Input: part model. Units: mm. Frame: model coordinates. Face numbers are marked on the shaded views. A direction names the side the tool comes from. Give positions to 0.01 mm unless a question says otherwise; leave off trailing zeros. Order: outer loops, then holes, each group sorted by start corner. A loop starts at its lowest first (then second) coordinate and runs counter-clockwise, first axis right, second up. Notation, with made-up numbers: (56.5, 64.5) - (69.5, 64.5) arc R11 ccw to (69.5, 76.5) - close; hole circle Ø2 at (-37, -38.75). An arc over 180 degrees is marked (long way). Use a Markdown table: item, result.
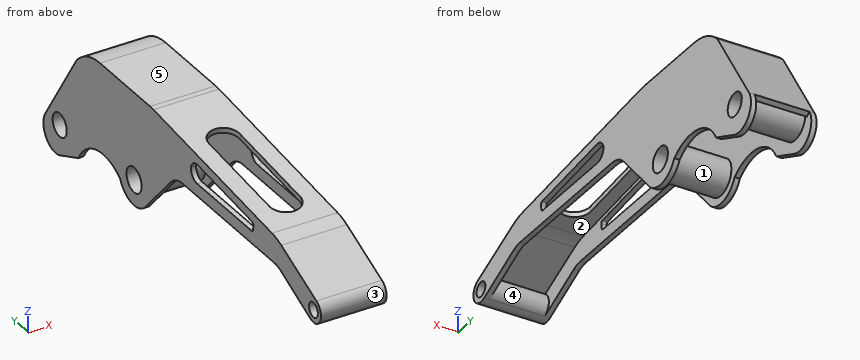
from build123d import *

# Parameters (mm, degrees)
F0_R        = 5.6533409101
F0_R_2      = 6.0582147302
F0_R_3      = 3.5468264326
F1_DEPTH    = 31.75
F2_T        = 2.54
F2_T3_DEPTH = 36.83
F4_DEPTH    = 25.4
F6_DEPTH    = 31.751
F7_T1_DEPTH = 2.54
F7_T3_DEPTH = 2.54
F8_R        = 1.27


# Not quite as in the source:
# - a fillet or chamfer that OpenCascade refuses, or shapes differently, is made with other operations: its cross-section is extruded or revolved along the edge and cut away or added
# - a shell that OpenCascade refuses in one call is made with other operations: the cavity is built on its own and cut out


with BuildPart() as f1:
    # F0 (on Right) → F1 (new body)
    with BuildSketch(Plane.YZ):
        with BuildLine():
            Line((-118.2969192854, 30.0553025028), (-146.4621126652, 17.7829619497))
            ThreePointArc((-146.4621126652, 17.7829619497), (-149.6721200055, 9.657338463), (-141.4359788777, 6.7425685756))
            Line((-141.4359788777, 6.7425685756), (-117.9046317908, 17.455203049))
            ThreePointArc((-117.9046317908, 17.455203049), (-115.3347971308, 18.3079832041), (-112.6425907814, 18.5966164392))
            Line((-112.6425907814, 18.5966164392), (-39.032237408, 18.5966164392))
            ThreePointArc((-39.032237408, 18.5966164392), (-33.875711062, 17.5026595222), (-29.6075339545, 14.4092520366))
            Line((-29.6075339545, 14.4092520366), (-10.1635284412, -7.1180392256))
            ThreePointArc((-10.1635284412, -7.1180392256), (1.0358015594, -12.3649063046), (11.2061193672, -5.3279153072))
            ThreePointArc((11.2061193672, -5.3279153072), (29.7519512617, -1.1293262164), (44.7507215315, -12.8174792531))
            Line((44.7507215315, -12.8174792531), (59.2673632914, -19.1176440206))
            ThreePointArc((59.2673632914, -19.1176440206), (70.5449926496, -16.490786447), (71.3009120761, -4.9359653548))
            Line((71.3009120761, -4.9359653548), (46.0699528524, 34.1704526075))
            ThreePointArc((46.0699528524, 34.1704526075), (37.5779975797, 40.2467968073), (27.3589767296, 42.3931602559))
            Line((27.3589767296, 42.3931602559), (-12.8688071267, 42.3931602559))
            ThreePointArc((-12.8688071267, 42.3931602559), (-14.2256285087, 42.3568949126), (-15.5785754345, 42.2482024399))
            Line((-15.5785754345, 42.2482024399), (-110.8605493232, 32.0248153133))
            ThreePointArc((-110.8605493232, 32.0248153133), (-114.6537287056, 31.3232183323), (-118.2969192854, 30.0553025028))
        make_face()
        with Locations((59.7972124815, -4.6163224615)):
            Circle(F0_R, mode=Mode.SUBTRACT)
        Circle(F0_R_2, mode=Mode.SUBTRACT)
        with Locations((-144.1483274102, 12.1720423922)):
            Circle(F0_R_3, mode=Mode.SUBTRACT)
    extrude(amount=F1_DEPTH)

    # F2: shell of thickness 2.54, made by hand


with BuildPart() as f2_core1:
    # F2_t2: copy of F1
    add(f1.part)

    # the walls: a layer under each face that stays
    f2_faces = [f2_core1.faces().sort_by_distance(p)[0] for p in [
        (15.875, -63.2195623789, 37.1365088766),
        (15.875, -114.6537287056, 31.3232183323),
        (15.875, -132.3795159753, 23.9191322262),
        (15.875, -149.6721200055, 9.657338463),
        (15.875, 58.6854324642, 14.6172436263),
        (15.875, 37.5779975797, 40.2467968073),
        (15.875, 7.2450848014, 42.3931602559),
        (15.875, -14.2256285087, 42.3568949126),
        (15.875, 54.1438715714, -4.6163224615),
        (15.875, -6.0582147302, 0),
        (15.875, -147.6951538428, 12.1720423922),
        (0, -38.6823777389, 32.0074819355),
        (31.75, -38.6823777389, 32.0074819355),
    ]]
    thicken(f2_faces, amount=-F2_T, mode=Mode.SUBTRACT)

    # F2_s4 → F2_t3 (cut)
    with BuildSketch(Plane.YZ.offset(-2.54)):
        Polygon((-146.4819420371, 17.8297292802), (-145.4474988382, 15.4544090123), (-145.4705469322, 15.4443663311), (-145.4937892966, 15.4347818344), align=None)
    extrude(amount=F2_T3_DEPTH, mode=Mode.SUBTRACT)


with BuildPart() as f1_1:
    add(f1.part)

    # what is left inside the walls is the cavity
    f2_cavity = [f2_core1.part.solids().sort_by_distance(p)[0] for p in [
        (29.1846, -87.664257, 19.92847),
    ]]
    add(f2_cavity, mode=Mode.SUBTRACT)

    # F3 (on face) → F4 (cut)
    with BuildSketch(Plane(origin=(0, -4.6587823298, 43.4198539884), x_dir=(1, 0, 0), z_dir=(0, -0.1066837916, 0.9942929994))):
        with BuildLine():
            Line((8.5797651154, -41.550964987), (8.5891456531, -90.6220046018))
            ThreePointArc((8.5891456531, -90.6220046018), (15.9863896259, -97.7322088228), (23.5313536211, -90.7789548531))
            Line((23.5313536211, -90.7789548531), (23.5313536211, -42.0811111897))
            ThreePointArc((23.5313536211, -42.0811111897), (16.3302504196, -34.0689910553), (8.5797651154, -41.550964987))
        make_face()
    extrude(amount=-F4_DEPTH, mode=Mode.SUBTRACT)

    # F5 (on face) → F6 (cut, through all)
    with BuildSketch(Plane.YZ.offset(31.75)):
        Polygon((-46.1267865209, 34.4621779106), (-96.0500612855, 29.1056036949), (-95.512650907, 24.6252825343), (-45.0713257087, 24.6252825343), align=None)
    extrude(amount=-F6_DEPTH, mode=Mode.SUBTRACT)

    # F7: fillet of radius 5.08 on 4 edges, made by hand

    # F7_s2 → F7_t1 (join)
    with BuildSketch(Plane.YZ.offset(29.21)):
        with BuildLine():
            ThreePointArc((-50.7255480205, 24.6252825343), (-46.9466907461, 26.3101922999), (-45.6745395837, 30.2472361958))
            Line((-45.6745395837, 30.2472361958), (-45.0713257087, 24.6252825343))
            Line((-45.0713257087, 24.6252825343), (-50.7255480205, 24.6252825343))
        make_face()
        with BuildLine():
            ThreePointArc((-51.1777949577, 33.920224249), (-47.4474580879, 32.8240372389), (-45.5848328594, 29.4111694737))
            Line((-45.5848328594, 29.4111694737), (-46.1267865209, 34.4621779106))
            Line((-46.1267865209, 34.4621779106), (-51.1777949577, 33.920224249))
        make_face()
    extrude(amount=F7_T1_DEPTH)

    # F7_s4 → F7_t3 (join)
    with BuildSketch(Plane.YZ):
        with BuildLine():
            ThreePointArc((-51.1777949577, 33.920224249), (-47.4474580879, 32.8240372389), (-45.5848328594, 29.4111694737))
            Line((-45.5848328594, 29.4111694737), (-46.1267865209, 34.4621779106))
            Line((-46.1267865209, 34.4621779106), (-51.1777949577, 33.920224249))
        make_face()
        with BuildLine():
            ThreePointArc((-50.7255480205, 24.6252825343), (-46.9466907461, 26.3101922999), (-45.6745395837, 30.2472361958))
            Line((-45.6745395837, 30.2472361958), (-45.0713257087, 24.6252825343))
            Line((-45.0713257087, 24.6252825343), (-50.7255480205, 24.6252825343))
        make_face()
    extrude(amount=F7_T3_DEPTH)

    # F8
    f8_edges = [f1_1.edges().sort_by_distance(p)[0] for p in [
        (30.48, -96.050061, 29.105604),
        (30.48, -95.512651, 24.625283),
        (1.27, -96.050061, 29.105604),
        (1.27, -95.512651, 24.625283),
    ]]
    fillet(f8_edges, radius=F8_R)


solid = f1_1.part
1. Section query D-D (y = 22.5). Return loops of the section in (x, z), then the cut area to 3 significant figures.
Response:
| item | result |
|---|---|
| outline | (0, -0.73) - (2.54, -0.73) - (2.54, 39.85) - (29.21, 39.85) - (29.21, -0.73) - (31.75, -0.73) - (31.75, 42.39) - (0, 42.39) - close |
| area | 287 mm^2 |
2. Set-up query: the marked faces 4 and 5. Return all of +Z, -Z, +X, -X, +Y, -Y with unobstructed straight access to the full face (end or side cutting, diameter ignored); none if empty.
Response:
| item | result |
|---|---|
| face 4 | none |
| face 5 | +Z, +X, -X, +Y, -Y |
3. Section query C-C (x = 26). Return loops of the section in (y, z), then the cut area to 3 significant figures.
Response:
| item | result |
|---|---|
| outline | (-146.46, 17.78) arc R6.07 ccw (long way) to (-141.44, 6.74) - (-141.17, 6.86) arc R6.09 ccw to (-141.01, 17.39) - (-117.28, 27.73) arc R22.86 cw to (-110.59, 29.5) - (-15.31, 39.72) arc R22.86 cw to (-12.87, 39.85) - (27.36, 39.85) arc R22.86 cw to (44.06, 32.61) - (63.29, 2.8) arc R8.19 ccw (long way) to (67.99, -4.49) - (69.17, -6.31) - (71.3, -4.94) - (46.07, 34.17) arc R25.4 ccw to (27.36, 42.39) - (-12.87, 42.39) arc R25.4 ccw to (-15.58, 42.25) - (-110.86, 32.02) arc R25.4 ccw to (-118.3, 30.06) - close; circle Ø17.2 at (0, 0); hole circle Ø7.09 at (-144.15, 12.17); hole circle Ø12.12 at (0, 0); hole circle Ø11.31 at (59.8, -4.62) |
| area | 905 mm^2 |
4. Mould query, pull axis Z, two halves, no side actions, for the marked faces 1, 2 and 3. Classes: pulls with the +Z half, pulls with the -Z half, needs draft (parallel to the pull), parting line crosses it, or undercut.
Response:
| item | result |
|---|---|
| face 1 | undercut |
| face 2 | pulls with the -Z half |
| face 3 | parting line crosses it |
5. Section query A-A (y = 0). Return loops of the section in (x, z).
Response:
| item | result |
|---|---|
| outline | (0, -12.41) - (2.54, -12.41) - (2.54, -8.6) - (29.21, -8.6) - (29.21, -12.41) - (31.75, -12.41) - (31.75, -6.06) - (0, -6.06) - close; (0, 6.06) - (31.75, 6.06) - (31.75, 42.39) - (0, 42.39) - close; hole (2.54, 8.6) - (29.21, 8.6) - (29.21, 39.85) - (2.54, 39.85) - close |
6. Section query B-B (x = 14.5). Return loops of the section in (y, z), then the cut area to 3 significant figures.
Response:
| item | result |
|---|---|
| outline | (-146.46, 17.78) arc R6.07 ccw (long way) to (-141.44, 6.74) - (-141.17, 6.86) arc R6.09 ccw to (-141.01, 17.39) - (-117.28, 27.73) arc R22.86 cw to (-110.59, 29.5) - (-101.4, 30.49) - (-101.67, 33.01) - (-110.86, 32.02) arc R25.4 ccw to (-118.3, 30.06) - close; (-38.69, 39.77) - (-38.42, 37.24) - (-15.31, 39.72) arc R22.86 cw to (-12.87, 39.85) - (27.36, 39.85) arc R22.86 cw to (44.06, 32.61) - (63.29, 2.8) arc R8.19 ccw (long way) to (67.99, -4.49) - (69.17, -6.31) - (71.3, -4.94) - (46.07, 34.17) arc R25.4 ccw to (27.36, 42.39) - (-12.87, 42.39) arc R25.4 ccw to (-15.58, 42.25) - close; circle Ø17.2 at (0, 0); hole circle Ø7.09 at (-144.15, 12.17); hole circle Ø12.12 at (0, 0); hole circle Ø11.31 at (59.8, -4.62) |
| area | 744 mm^2 |
7. Pin query (flat end, axial travel): pin 1 (4 mm diameter, centred on x = 8.5, z = -8, fed in from -Y); pin 2 (12 mm diameter, centred on y = -87.5, z = 7, fed in from -X); pin 3 (8 mm diameter, centred on x = 5.5, y = -42, fed in from -Z); pin 4 (1.5 mm diameter, centred on x = 17, y = 22.5, fed in from -Z). Return the tip coordinate at first contact, or that it passes through.
Response:
| item | result |
|---|---|
| pin 1 | stops at y = -6.16 |
| pin 2 | passes through |
| pin 3 | stops at z = 18.6 |
| pin 4 | stops at z = 39.85 |
8. Material intervals for line 1 along Z through (x, y) = (20, 0); line 2 along X through (y, z) = (-35, 24); line 3 along Z through (x, y) = (22.5, 61.5), sorted ascending.
Response:
| item | result |
|---|---|
| line 1 | z = -8.6 to -6.06, 6.06 to 8.6, 39.85 to 42.39 |
| line 2 | x = 0 to 2.54, 29.21 to 31.75 |
| line 3 | z = -12.63 to -10.01, 0.77 to 3.4, 5.57 to 10.25 |
